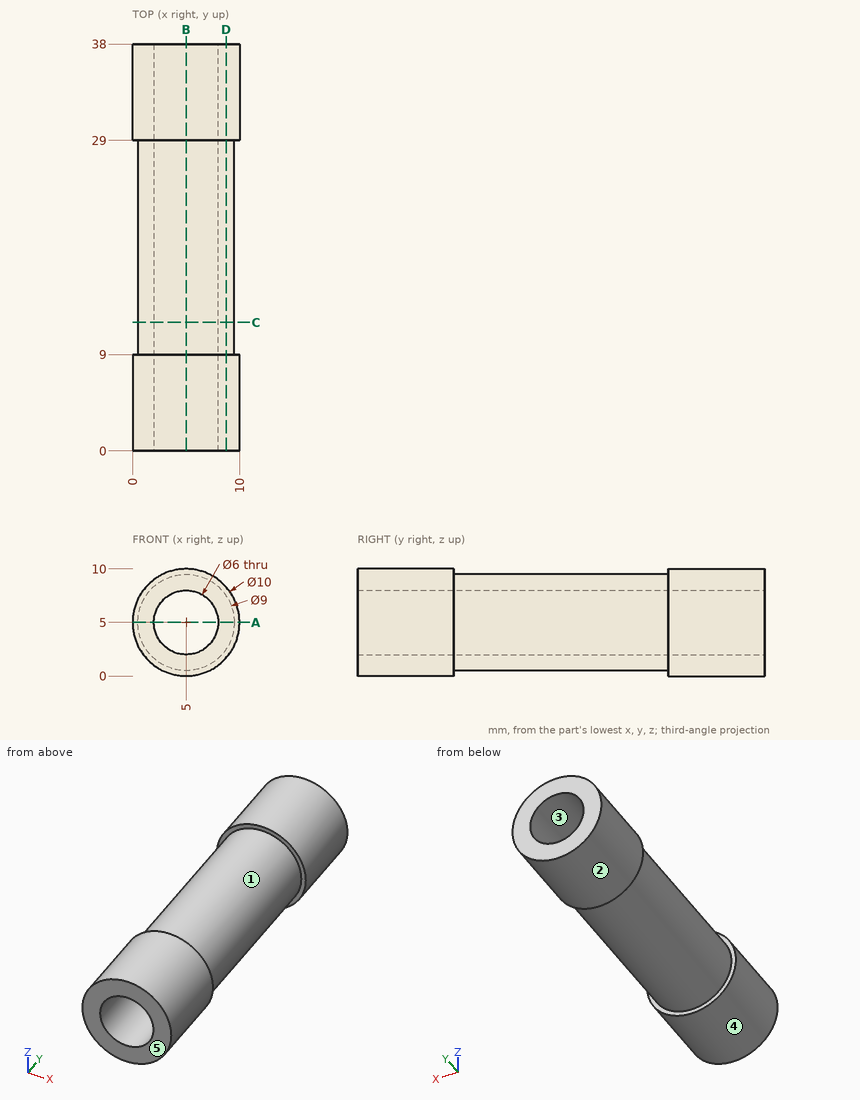
Could you check a few things on this drawing? It's one solid part, dimensions in mm from its lowest x, y, z. A direction names the side the tool comes from. Coordinates: 2 decimals unless noted, no trailing zeros. Order: outer loops, then holes, each group sorted by start corner. A loop starts at its lowest first (then second) coordinate and runs counter-clockwise, first axis right, second up.
1) Imagine slicing it at C-C on y = 12. List the corners of the cut face in (x, z) for me, and give its area (3 significant figures).
2) I need wall thicknesses on line 1 (Y direction, x = 6.5, z = 9.5); line 2 (Z direction, x = 5, y = 16.5); line 3 (Z direction, x = 6.75, y = 23.5). Which ranges of each line are inside material? Lowest first, please.
3) Imagine slicing it at A-A on z = 5. List the corners of the cut face in (x, y) for me, and give its area (3 significant figures).
4) Imagine slicing it at D-D on x = 8.75. List the corners of the cut face in (y, z) for me.
5) Will these pins go through, and if not, where does the flat tip stop? pin 1 (6 mm diameter, centred on x = 7, y = 15.5, fed in from +Z); pin 2 (1 mm diameter, centred on y = 30, z = 2.5, fed in from +X); pin 3 (4 mm diameter, centred on x = 7, y = 10, fed in from +Z).
6) Imagine slicing it at B-B on x = 5. List the corners of the cut face in (y, z) for me, and give its area (3 significant figures).
7) Which directions (+Z, -Z, +X, -X, +Y, -Y) give clear straight access to the entire face, cutting with the end or side of a thin tool? Please do the marked faces 1 and 2.
8) We'd pull the mould along X, two halves only. Please class the marked faces 3, 4 and 5: +X half, -X half, draft (parallel to the pull), parting line (faces both ways), or undercut.
Response values:
1. outline: circle Ø9 at (5, 5); hole circle Ø6 at (5, 5)
1. area: 35.3 mm2
2. line 1: y = 0 to 9, 29 to 38
2. line 2: z = 0.5 to 2, 8 to 9.5
2. line 3: z = 0.85 to 2.56, 7.44 to 9.15
3. outline: (0, 0) - (2, 0) - (2, 38) - (0, 38) - (0, 29) - (0.5, 29) - (0.5, 9) - (0, 9) - close; (8, 0) - (10, 0) - (10, 9) - (9.5, 9) - (9.5, 29) - (10, 29) - (10, 38) - (8, 38) - close
3. area: 132 mm2
4. outline: (0, 1.69) - (9, 1.69) - (9, 2.51) - (29, 2.51) - (29, 1.69) - (38, 1.69) - (38, 8.31) - (29, 8.31) - (29, 7.49) - (9, 7.49) - (9, 8.31) - (0, 8.31) - close
5. pin 1: stops at z = 9.5
5. pin 2: stops at x = 9.58
5. pin 3: stops at z = 9.99
6. outline: (0, 0) - (9, 0) - (9, 0.5) - (29, 0.5) - (29, 0) - (38, 0) - (38, 2) - (0, 2) - close; (0, 8) - (38, 8) - (38, 10) - (29, 10) - (29, 9.5) - (9, 9.5) - (9, 10) - (0, 10) - close
6. area: 132 mm2
7. face 1: none
7. face 2: +Y, -Y
8. face 3: undercut
8. face 4: parting line
8. face 5: draft
